```python
from build123d import *
from OCP.BRepFilletAPI import BRepFilletAPI_MakeChamfer

# Parameters (mm, degrees)
SKETCH1_W           = 1.5
SKETCH1_H           = 4
BOSS_EXTRUDE2_DEPTH = 5
FILLET1_R           = 0.5
CHAMFER1_SIZE       = 0.3
CHAMFER1_SIZE2      = 5.724341006
FILLET2_R           = 1


with BuildPart() as part:
    # Sketch1 → Boss-Extrude2 (new body)
    with BuildSketch(Plane.XY):
        with BuildLine():
            Line((-18, 0), (-18, -45))
            Line((-18, -45), (-13, -45))
            Line((-13, -45), (-13, 0))
            Line((-13, 0), (-14, 0))
            ThreePointArc((-14, 0), (-17.356723571, 5.717389506), (-22, 10.449843403))
            ThreePointArc((-22, 10.449843403), (-25.217580201, 14.024096355), (-27.099300045, 18.449843403))
            ThreePointArc((-27.099300045, 18.449843403), (-30.501361107, 62.323372475), (-20, 105.057223081))
            ThreePointArc((-20, 105.057223081), (-16.767609995, 109.972410851), (-12, 113.418758324))
            ThreePointArc((-12, 113.418758324), (-8.588186354, 114.5997714), (-5, 115))
            Line((-5, 115), (0, 115))
            Line((0, 115), (5, 115))
            ThreePointArc((5, 115), (8.588186354, 114.5997714), (12, 113.418758324))
            ThreePointArc((12, 113.418758324), (16.767609995, 109.972410851), (20, 105.057223081))
            ThreePointArc((20, 105.057223081), (30.501361107, 62.323372475), (27.099300045, 18.449843403))
            ThreePointArc((27.099300045, 18.449843403), (25.217580201, 14.024096355), (22, 10.449843403))
            ThreePointArc((22, 10.449843403), (17.356723571, 5.717389506), (14, 0))
            Line((14, 0), (13, 0))
            Line((13, 0), (13, -45))
            Line((13, -45), (18, -45))
            Line((18, -45), (18, 0))
            Line((18, 0), (20, 0))
            ThreePointArc((20, 0), (22.171979479, 3.570426989), (25.114361701, 6.538225938))
            ThreePointArc((25.114361701, 6.538225938), (29.4338834, 11.336571968), (31.960045669, 17.278027726))
            ThreePointArc((31.960045669, 17.278027726), (35.484647146, 62.731857791), (24.605032643, 107.004958781))
            ThreePointArc((24.605032643, 107.004958781), (20.380385499, 113.428977522), (14.149246958, 117.933261343))
            ThreePointArc((14.149246958, 117.933261343), (9.667432642, 119.743515679), (5, 121))
            Line((5, 121), (-5, 121))
            ThreePointArc((-5, 121), (-9.667432642, 119.743515679), (-14.149246958, 117.933261343))
            ThreePointArc((-14.149246958, 117.933261343), (-20.380385499, 113.428977522), (-24.605032643, 107.004958781))
            ThreePointArc((-24.605032643, 107.004958781), (-35.484647146, 62.731857791), (-31.960045669, 17.278027726))
            ThreePointArc((-31.960045669, 17.278027726), (-29.4338834, 11.336571968), (-25.114361701, 6.538225938))
            ThreePointArc((-25.114361701, 6.538225938), (-22.171979479, 3.570426989), (-20, 0))
            Line((-20, 0), (-18, 0))
        make_face()
        with Locations((15.5, -8)):
            Rectangle(SKETCH1_W, SKETCH1_H, mode=Mode.SUBTRACT)
        with Locations((-15.5, -40)):
            Rectangle(SKETCH1_W, SKETCH1_H, mode=Mode.SUBTRACT)
        with Locations((15.5, -40)):
            Rectangle(SKETCH1_W, SKETCH1_H, mode=Mode.SUBTRACT)
        with Locations((-15.5, -8)):
            Rectangle(SKETCH1_W, SKETCH1_H, mode=Mode.SUBTRACT)
        with Locations((-15.5, -30)):
            Rectangle(SKETCH1_W, SKETCH1_H, mode=Mode.SUBTRACT)
        with Locations((15.5, -30)):
            Rectangle(SKETCH1_W, SKETCH1_H, mode=Mode.SUBTRACT)
    extrude(amount=BOSS_EXTRUDE2_DEPTH)

    # Fillet1
    fillet1_edges = [part.edges().sort_by_distance(p)[0] for p in [
        (-20, 0, 2.5),
        (20, 0, 2.5),
        (13, 0, 2.5),
        (14, 0, 2.5),
        (-14, 0, 2.5),
        (-13, 0, 2.5),
    ]]
    fillet(fillet1_edges, radius=FILLET1_R)

    # Chamfer1: one chamfer whose edges measure the first distance from different faces: ONE call of the kernel's chamfer builder (chamfer() names one face for all edges)
    chamfer1_edges_1 = [part.edges().sort_by_distance(p)[0] for p in [
        (-18, 0, 2.5),
    ]]
    chamfer1_side_1 = [part.faces().sort_by_distance(p)[0] for p in [
        (-18.841037528, 0, 2.5),
    ]]
    chamfer1_edges_2 = [part.edges().sort_by_distance(p)[0] for p in [
        (18, 0, 2.5),
    ]]
    chamfer1_side_2 = [part.faces().sort_by_distance(p)[0] for p in [
        (18.841037528, 0, 2.5),
    ]]
    chamfer1 = BRepFilletAPI_MakeChamfer(part.part.solid().wrapped)
    for e in chamfer1_edges_1:
        chamfer1.Add(CHAMFER1_SIZE, CHAMFER1_SIZE2, e.wrapped, chamfer1_side_1[0].wrapped)  # the first distance lies on this face
    for e in chamfer1_edges_2:
        chamfer1.Add(CHAMFER1_SIZE, CHAMFER1_SIZE2, e.wrapped, chamfer1_side_2[0].wrapped)  # the first distance lies on this face
    add(Compound.cast(chamfer1.Shape()), mode=Mode.REPLACE)

    # Fillet2
    fillet2_edges = [part.edges().sort_by_distance(p)[0] for p in [
        (-13, -45, 2.5),
        (-18, -45, 2.5),
        (18, -45, 2.5),
        (13, -45, 2.5),
    ]]
    fillet(fillet2_edges, radius=FILLET2_R)


solid = part.part
```
Geometry: final body of the model. Coordinates: model frame, mm. A direction names the side the tool comes from. Round coordinates to 2 decimals unless told otherwise and drop trailing zeros. Order: outer loops, then holes, each group sorted by start corner. A loop starts at its lowest first (then second) coordinate and runs counter-clockwise, first axis right, second up. Notation, with made-up numbers: (65, -11.5) - (86, -11.5) arc R24 ccw to (86, 1.5) - close; hole circle Ø8 at (55, 84). An arc over 180 degrees is marked (long way). Write item = value, one per line. Start each with the question number.
Q1. Cut plane B-B on y = 20. Return the cut outline in (x, z), and give its area (3 significant figures).
Q2. Pull-direction query (X, two-part tool) for faces 4 (the flat face through (14.75, -40, 2)), 5 (the cylindrical face through (-20.305, 113.507, 2.465)), 6 (the cylindrical face through (29.385, 11.26, 2.465)); classes: +X half, -X half, draft (parallel to the pull), parting line (faces both ways), or undercut.
Q3. Pin query (flat end, axial travel): pin 1 (2 mm diameter, centred on x = -14.5, z = 4, fed in from +Y); pin 2 (2.5 mm diameter, centred on y = -31, z = 2.5, fed in from -X); pin 3 (12 mm diameter, centred on x = 14, y = 103, fed in from -Z); pin 4 (0.7 mm diameter, centred on x = -19, z = 3, fed in from -Y). Return the tip coordinate at first contact, or that it passes through.
Q4. Cut plane C-C on z = 2.8. Give the number of separate pieces and of enclosed holes in the cut face, and give its area (3 significant figures).
Q5. Ray query, line 1 (X direction, y = 50, z = 0.65); line 2 (X direction, y = 41, z = 2); line 3 (Y direction, x = 17, z = 3.25). Return the intervals inside material, ascending. Write a range as from..to.
Q6. Cut plane A-A on x = -29. Return the cut outline in (y, z), and give its area (3 significant figures).
Q7. Access query for faces 1 (the cylindrical face through (35.536, 62.093, 2.465)), 2 (the flat face through (-18, -25, 2)), 3 (the cylindrical face through (16.71, 110.03, 2.46)). Directions: +Z, -Z, +X, -X, +Y, -Y. A direction counts if a zero-diameter tool reaches every point of the face in a straight line with its end or side. Return the directions, or none.
Q8. Cut plane D-D on x = 1. Return the cut outline in (y, z), and give its area (3 significant figures).
Outcome:
q1.outline = (-32.59, 0) - (-27.46, 0) - (-27.46, 5) - (-32.59, 5) - close; (27.46, 0) - (32.59, 0) - (32.59, 5) - (27.46, 5) - close
q1.area = 51.2 mm^2
q2.face_4 = undercut
q2.face_5 = -X half
q2.face_6 = +X half
q3.pin_1 = 118.24
q3.pin_2 = -18
q3.pin_3 = through
q3.pin_4 = 0
q4.separate_pieces = 1
q4.enclosed_holes = 6
q4.area = 1,830 mm^2
q5.line_1 = -35.96..-30.96, 30.96..35.96
q5.line_2 = -35.62..-30.61, 30.61..35.62
q5.line_3 = -45..5.24, 109.72..116.29
q6.outline = (10.68, 0) - (27.71, 0) - (27.71, 5) - (10.68, 5) - close; (74.26, 0) - (95.2, 0) - (95.2, 5) - (74.26, 5) - close
q6.area = 190 mm^2
q7.face_1 = +Z, -Z, +X
q7.face_2 = +Z, -Z, -X, -Y
q7.face_3 = +Z, -Z
q8.outline = (115, 0) - (121, 0) - (121, 5) - (115, 5) - close
q8.area = 30.0 mm^2
